```python
from build123d import *

# Parameters (mm, degrees)
F0_W      = 111.252
F0_H      = 19.05
F1_DEPTH  = 33.274
F3_DEPTH  = 111.253
F5_ANGLE  = 45
F7_DEPTH  = 35.56
F9_DEPTH  = 98.2604240246
F11_DEPTH = 60.96
F13_DEPTH = 6.35


with BuildPart() as f1:
    # F0 (on Front) → F1 (new body, symmetric)
    with BuildSketch(Plane.XZ):
        with Locations((-55.626, -9.525)):
            Rectangle(F0_W, F0_H)
    extrude(amount=F1_DEPTH, both=True)

    # F2 (on Right) → F3 (cut, through all)
    with BuildSketch(Plane.YZ):
        Polygon((-11.3380621702, -19.05), (11.3380621702, -19.05), (16.764, -9.652), (-16.764, -9.652), align=None)
    extrude(amount=-F3_DEPTH, mode=Mode.SUBTRACT)

    # F4 (on Top) → F5 (revolve)
    with BuildSketch(Plane.XY):
        Polygon((-78.2938633586, -9.144), (-47.498, -26.924), (-40.386, -14.6056546566), (-71.1818633586, 3.1743453434), align=None)
    revolve(axis=Axis((-62.8959316793, -18.034, 0), (0.8660254038, -0.5, 0)), revolution_arc=F5_ANGLE)

    # F6 (on face) → F7 (join)
    with BuildSketch(Plane(origin=(-23.9650660143, 13.8362373145, 0), x_dir=(0.5, 0.8660254038, 0), z_dir=(0.8660254038, -0.5, 0))):
        Polygon((17.5919761002, 64.6578440717), (-47.0658679715, 0), (-32.8418679715, 0), (31.8159761002, 64.6578440717), align=None)
    extrude(amount=-F7_DEPTH)

    # F8 (on face) → F9 (cut, through all)
    with BuildSketch(Plane(origin=(-23.9650660143, 13.8362373145, 0), x_dir=(0.5, 0.8660254038, 0), z_dir=(0.8660254038, -0.5, 0))):
        Polygon((31.8159761002, 64.6578440717), (17.5919761002, 64.6578440717), (24.7039761002, 57.5458440717), align=None)
    extrude(amount=-F9_DEPTH, mode=Mode.SUBTRACT)

    # F10 (on face) → F11 (cut)
    with BuildSketch(Plane(origin=(20.562455043, 35.6152168628, 41.124910086), x_dir=(0.9354143467, -0.2314550249, -0.2672612419), z_dir=(0.3535533906, 0.6123724357, 0.7071067812))):
        Polygon((-42.8532903043, -11.5935840247), (-61.6659547317, -3.9133459332), (-60.671811363, -11.1779871697), (-48.6475824802, -16.0868580553), align=None)
    extrude(amount=-F11_DEPTH, mode=Mode.SUBTRACT)

    # F12 (on face) → F13 (cut)
    with BuildSketch(Plane(origin=(-11.7664669929, -20.3801186572, 23.5329339857), x_dir=(0.9354143467, -0.2314550249, 0.2672612419), z_dir=(-0.3535533906, -0.6123724357, 0.7071067812))):
        with BuildLine():
            Line((-37.1272253429, 12.1321385858), (-49.1514542257, 17.0410094713))
            ThreePointArc((-49.1514542257, 17.0410094713), (-45.5937752271, 8.5744595872), (-37.1272253429, 12.1321385858))
        make_face()
    extrude(amount=-F13_DEPTH, mode=Mode.SUBTRACT)


solid = f1.part
```
Here's how the part is built. I have some questions about the finished solid (model axes, mm). A direction names the side the tool comes from. Coordinates: 2 decimals unless noted, no trailing zeros. Write each loop counter-clockwise with the first axis right and the second up, starting at its lowest first coordinate (ties: lowest second). Pieces come first, ordered by that corner, then holes. Notation, with made-up numbers: (7.25, 38) -> (27.25, 38) arc R14 ccw to (27.25, 45) -> close; hole circle Ø7 at (-23, -36.5). An arc over 180 degrees is marked (long way). Use a Markdown table: item, result. Add a question column.
(1) If we section it at B-B, the plane y = -23.5: Write out the boundary of the cut face in (x, z).
(2) If we section it at A-A, the plane x = -30: Write out the boundary of the cut face in (y, z), and give its area (3 significant figures).
(3) If we section it at C-C, the plane z = 51: Write out the boundary of the cut face in (x, y), and give its area (3 significant figures).
(4) For faces 1 (the flat face through (-28.31, 6.31, 30.09)), 2 (the flat face through (-41.38, 18.73, 28.37)), 3 (the flat face through (-44, -0.67, 18.62)), which set-ups out of +Z, -Z, +X, -X, +Y, -Y let a thin tool reach every point of the face, with its end or its side?
(5) We'd pull the mould along X, two halves only. Please class faces 4 (the flat face through (-111.252, 0, -8)), 5 (the flat face through (-56, 33.274, -9)), 6 (the flat face through (-57.461, 7.202, 18.532)): +X half, -X half, draft (parallel to the pull), parting line (faces both ways), or undercut.
(6) If we section it at D-D, the plane y = 21.5: Write out the boundary of the cut face in (x, z), and give its area (3 significant figures).
(7) Please list where these lines run through material, in increasing order: line 1 (Z direction, x = -23, y = -8); line 2 (Z direction, x = -85, y = 23); line 3 (Z direction, x = -15, y = -14.5).
(8) I'm going to push flat-ended pins straight in: P1, Ø21, axis at x = -46.5, z = -8.5, coming from the +Y side; P2, Ø8, axis at x = -54.5, z = 19, coming from the -Y side; P3, Ø10, axis at x = -97, y = 7.5, coming from the -Z side; P4, Ø4, axis at x = -37, y = 16, coming from the +Z side. Where does each tip first touch, or does it pass through?
Outcome:
| question | item | result |
|---|---|---|
| 1 | outline | (-111.25, -19.05) -> (0, -19.05) -> (0, 0) -> (-45.52, 0) -> (-45.52, 3.95) -> (-53.43, 0) -> (-111.25, 0) -> close |
| 2 | outline | (-33.27, -19.05) -> (-11.34, -19.05) -> (-16.76, -9.65) -> (16.76, -9.65) -> (11.34, -19.05) -> (33.27, -19.05) -> (33.27, 0) -> (-33.27, 0) -> close; (3.38, 20.77) -> (45.85, 57.55) -> (42.82, 60.17) -> (18.62, 39.21) -> (25.96, 54.54) -> (3.38, 35) -> close |
| 2 | area | 1,390 mm^2 |
| 3 | outline | (-52.79, 35.02) -> (-43.02, 29.38) -> (-41.7, 38.99) -> (-24.11, 28.83) -> (-31.77, 22.89) -> (-22, 17.24) -> (-14.89, 29.56) -> (-45.68, 47.34) -> close |
| 3 | area | 356 mm^2 |
| 4 | face 1 | +Z, +X, -Y |
| 4 | face 2 | +X, +Y |
| 4 | face 3 | none |
| 5 | face 4 | -X half |
| 5 | face 5 | draft |
| 5 | face 6 | undercut |
| 6 | outline | (-111.25, -19.05) -> (0, -19.05) -> (0, 0) -> (-111.25, 0) -> close; (-60.6, 21.16) -> (-19.54, 41.69) -> (-19.54, 55.92) -> (-32.57, 49.4) -> (-28.34, 42.54) -> (-51.8, 30.8) -> (-47.57, 41.9) -> (-60.6, 35.38) -> close |
| 6 | area | 2,530 mm^2 |
| 7 | line 1 | z = -9.65 to 0 |
| 7 | line 2 | z = -19.05 to 0 |
| 7 | line 3 | z = -19.05 to -13.57, -9.65 to 0 |
| 8 | P1 | stops at y = 33.27 |
| 8 | P2 | stops at y = -6.11 |
| 8 | P3 | stops at z = -19.05 |
| 8 | P4 | stops at z = 44.1 |
